Drawing for the job (mm, zero at the part's lowest x, y, z). Coordinates: 2 decimals unless noted, no trailing zeros. Write each loop counter-clockwise with the first axis right and the second up, starting at its lowest first coordinate (ties: lowest second). Pieces come first, ordered by that corner, then holes. Notation, with made-up numbers: (85.5, 82.5) -> (111.5, 82.5) arc R26 ccw to (111.5, 116.5) -> close; hole circle Ø5 at (18, 23.25). An arc over 180 degrees is marked (long way). Answer as CSV lines item,"result".
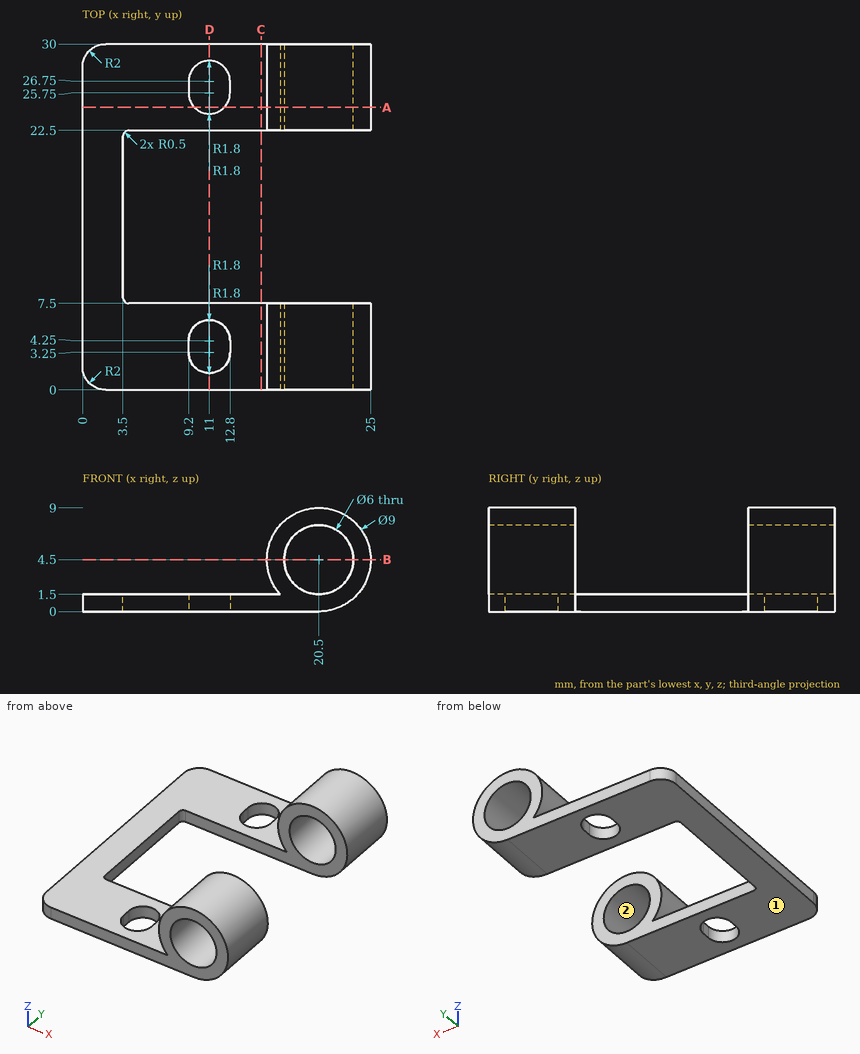
Item 1: Wall check: line 1 (Z direction, x = 20.5, y = 26.25); line 2 (X direction, y = 25.75, z = 4.5); line 3 (Y direction, x = 22, z = 1.5). Give the ranges that are in metal, low to high. Write a range as from..to.
Answer below:
line 1,"z = 0..1.5, 7.5..9"
line 2,"x = 16..17.5, 23.5..25"
line 3,"y = 0..7.5, 22.5..30"
Item 2: Saw through at B-B on z = 4.5. Give the cut face in (x, y), and give its area (3 significant figures).
Answer below:
outline,"(16, 0) -> (17.5, 0) -> (17.5, 7.5) -> (16, 7.5) -> close; (16, 22.5) -> (17.5, 22.5) -> (17.5, 30) -> (16, 30) -> close; (23.5, 0) -> (25, 0) -> (25, 7.5) -> (23.5, 7.5) -> close; (23.5, 22.5) -> (25, 22.5) -> (25, 30) -> (23.5, 30) -> close"
area,"45.0 mm2"
Item 3: Saw through at A-A on y = 24.5. Give the cut face in (x, z).
Answer below:
outline,"(0, 0) -> (9.7, 0) -> (9.7, 1.5) -> (0, 1.5) -> close; (12.3, 0) -> (20.5, 0) arc R4.5 ccw (long way) to (17.15, 1.5) -> (12.3, 1.5) -> close; hole circle Ø6 at (20.5, 4.5)"
Item 4: Flat gauge pins, fed straight in: pin 1 (3.5 mm diameter, centred on x = 20.5, z = 4.5, fed in from +Y); pin 2 (1.6 mm diameter, centred on y = 16.5, z = 0.5, fed in from +X); pin 3 (4 mm diameter, centred on y = 25, z = 5, fed in from -X); pin 4 (0.8 mm diameter, centred on y = 26, z = 1, fed in from +X). Where does each tip first touch, or does it go through?
Answer below:
pin 1,"passes through"
pin 2,"stops at x = 3.5"
pin 3,"stops at x = 16"
pin 4,"stops at x = 23.76"
Item 5: Saw through at C-C on x = 15.5. Give the cut face in (y, z).
Answer below:
outline,"(0, 0) -> (7.5, 0) -> (7.5, 1.5) -> (0, 1.5) -> close; (22.5, 0) -> (30, 0) -> (30, 1.5) -> (22.5, 1.5) -> close"
Item 6: Saw through at D-D on x = 11. Give the cut face in (y, z).
Answer below:
outline,"(0, 0) -> (1.45, 0) -> (1.45, 1.5) -> (0, 1.5) -> close; (6.05, 0) -> (7.5, 0) -> (7.5, 1.5) -> (6.05, 1.5) -> close; (22.5, 0) -> (23.95, 0) -> (23.95, 1.5) -> (22.5, 1.5) -> close; (28.55, 0) -> (30, 0) -> (30, 1.5) -> (28.55, 1.5) -> close"
Item 7: Two-plate mould, pull along Z, no slides. Class the marked faces 1 and 2: pulls with the +Z half, pulls with the -Z half, needs draft (parallel to the pull), parting line crosses it, or undercut.
Answer below:
face 1,"pulls with the -Z half"
face 2,"undercut"
